Here's how the part is built. I have some questions about the finished solid (model axes, mm). A direction names the side the tool comes from. Give positions to 0.01 mm unless a question says otherwise; leave off trailing zeros. Loops run counter-clockwise (first coordinate to the right, second up) from the corner with the lowest first, then second, coordinate; pieces in that order, holes last. Notation, with made-up numbers: (74, 80) - (92, 80) arc R10 ccw to (92, 88) - close; hole circle Ø2 at (-9.5, 42.25). An arc over 180 degrees is marked (long way). Use a Markdown table: item, result.
from build123d import *

# Parameters (mm, degrees)
SKETCH2_R           = 38.1
BOSS_EXTRUDE1_DEPTH = 76.2
SKETCH3_R           = 19.05
CUT_EXTRUDE1_DEPTH  = 76.2
FILLET1_R           = 2.54
BOSS_EXTRUDE2_DEPTH = 12.7
SKETCH5_R           = 1.778
CUT_EXTRUDE2_DEPTH  = 25.4
CIRPATTERN2_COUNT   = 4


with BuildPart() as part:
    # Sketch2 → Boss-Extrude1 (new body)
    with BuildSketch(Plane(origin=(0, 0, 0), x_dir=(1, 0, 0), z_dir=(0, 1, 0))):
        with Locations(Location((0, 0, 0), (0, 0, 90))):
            Circle(SKETCH2_R)
    extrude(amount=BOSS_EXTRUDE1_DEPTH)

    # Sketch3 → Cut-Extrude1 (cut)
    with BuildSketch(Plane(origin=(0, 76.2, 0), x_dir=(1, 0, 0), z_dir=(0, 1, 0))):
        with Locations(Location((0, 0, 0), (0, 0, 270))):
            Circle(SKETCH3_R)
    extrude(amount=-CUT_EXTRUDE1_DEPTH, mode=Mode.SUBTRACT)

    # Fillet1
    fillet1_edges = [part.edges().sort_by_distance(p)[0] for p in [
        (0, 76.2, 38.1),
    ]]
    fillet(fillet1_edges, radius=FILLET1_R)

    # Sketch4 → Boss-Extrude2 (add)
    with BuildSketch(Plane(origin=(0, 0, 0), x_dir=(1, 0, 0), z_dir=(0, 1, 0))):
        with BuildLine():
            Line((-37.567106623, 6.35), (-50.267106623, 6.35))
            Line((-50.267106623, 6.35), (-50.267106623, -6.35))
            Line((-50.267106623, -6.35), (-37.567106623, -6.35))
            ThreePointArc((-37.567106623, -6.35), (-38.1, 0), (-37.567106623, 6.35))
        make_face()
    boss_extrude2 = extrude(amount=BOSS_EXTRUDE2_DEPTH)

    # Sketch5 → Cut-Extrude2 (cut)
    with BuildSketch(Plane.XY.offset(6.35)):
        with Locations((-43.917106623, 6.35)):
            Circle(SKETCH5_R)
    cut_extrude2 = extrude(amount=-CUT_EXTRUDE2_DEPTH, mode=Mode.SUBTRACT)

    # CirPattern2: Boss-Extrude2, Cut-Extrude2 ×4 about axis
    cirpattern2_axis = Axis((0, 0, 0), (0, 1, 0))
    add([boss_extrude2.rotate(cirpattern2_axis, i * 360 / CIRPATTERN2_COUNT) for i in range(1, CIRPATTERN2_COUNT)])
    add([cut_extrude2.rotate(cirpattern2_axis, i * 360 / CIRPATTERN2_COUNT) for i in range(1, CIRPATTERN2_COUNT)], mode=Mode.SUBTRACT)


solid = part.part
(1) On a 3-axis mill with a long thin cutter (end or side, diameter ignored), from which of +Z, -Z, +X, -X, +Y, -Y can I reach the whole of each face in a straight line? I mean faces 1 (the face through (45, 8, -6.35)), 2 (the face through (0, 6, 50.267)), 3 (the face through (-45, 8, 6.35)), 4 (the face through (14.593, 36.314, -35.195)), 5 (the face through (-6.35, 8, -45)). Say none if no direction works.
A:
| item | result |
|---|---|
| face 1 | -Z, +X, +Y, -Y |
| face 2 | +Z, +X, -X, +Y, -Y |
| face 3 | +Z, -X, +Y, -Y |
| face 4 | +Y |
| face 5 | -Z, -X, +Y, -Y |
(2) Suppose I cut it at D-D on y = 63. Write out the boundary of the cut face in (x, z).
A:
| item | result |
|---|---|
| outline | circle Ø76.2 at (0, 0); hole circle Ø38.1 at (0, 0) |
(3) We'd pull the mould along X, two halves only. Please class faces 6 (the face through (-44, 12.7, 0)), 7 (the face through (42.275, 5.669, -0.089)), 8 (the face through (-11.59, 38.63, -15.12)), 9 (the face through (6.35, 8, 45)): pulls with the +X half, pulls with the -X half, needs draft (parallel to the pull), parting line crosses it, or undercut.
A:
| item | result |
|---|---|
| face 6 | needs draft |
| face 7 | undercut |
| face 8 | undercut |
| face 9 | pulls with the +X half |
(4) If I drill on line 1 (X direction, y = 43, z = 0); line 2 (Z direction, x = -16, y = 23); line 3 (Z direction, x = 9, y = 58), over which ranges is the centre line in solid material (lowest first)?
A:
| item | result |
|---|---|
| line 1 | -38.1 to -19.05, 19.05 to 38.1 |
| line 2 | -34.58 to -10.34, 10.34 to 34.58 |
| line 3 | -37.02 to -16.79, 16.79 to 37.02 |
(5) Suppose I cut it at A-A on y = 6.35. Count the separate pieces of the cut face and the enclosed holes in it, plus the area to 3 significant figures.
A:
| item | result |
|---|---|
| separate pieces | 5 |
| enclosed holes | 1 |
| area | 3,870 mm2 |
(6) Suppose I cut it at C-C on z = 0. Write out the boundary of the cut face in (x, y), plus the area to 3 significant figures.
A:
| item | result |
|---|---|
| outline | (-50.27, 0) - (-19.05, 0) - (-19.05, 76.2) - (-35.56, 76.2) arc R2.54 ccw to (-38.1, 73.66) - (-38.1, 12.7) - (-50.27, 12.7) - close; (19.05, 0) - (50.27, 0) - (50.27, 12.7) - (38.1, 12.7) - (38.1, 73.66) arc R2.54 ccw to (35.56, 76.2) - (19.05, 76.2) - close; hole circle Ø3.56 at (-43.92, 6.35); hole circle Ø3.56 at (43.92, 6.35) |
| area | 3,190 mm2 |
(7) Will these pins go through, and if not, where does the flat tip stop? pin 1 (4 mm diameter, centred on x = -1.5, z = 41.5, fed in from +Y); pin 2 (4 mm diameter, centred on y = 9, z = -44, fed in from -X); pin 3 (2 mm diameter, centred on y = 16.5, z = -12.5, fed in from +X).
A:
| item | result |
|---|---|
| pin 1 | y = 12.7 |
| pin 2 | x = -6.35 |
| pin 3 | x = 36.32 |
(8) Suppose I cut it at B-B on x = 0. Write out the boundary of the cut face in (y, z).
A:
| item | result |
|---|---|
| outline | (0, -50.27) - (12.7, -50.27) - (12.7, -38.1) - (73.66, -38.1) arc R2.54 ccw to (76.2, -35.56) - (76.2, -19.05) - (0, -19.05) - close; (0, 19.05) - (76.2, 19.05) - (76.2, 35.56) arc R2.54 ccw to (73.66, 38.1) - (12.7, 38.1) - (12.7, 50.27) - (0, 50.27) - close; hole circle Ø3.56 at (6.35, -43.92); hole circle Ø3.56 at (6.35, 43.92) |
